from build123d import *

# Parameters (mm, degrees)
F0_W      = 80
F0_H      = 42
F1_DEPTH  = 18
F2_W      = 50
F2_H      = 42
F3_DEPTH  = 30
F4_R      = 7
F5_DEPTH  = 48
F6_R      = 15
F7_DEPTH  = 42
F9_W      = 8.9407891482
F9_H      = 20
F10_DEPTH = 29
F11_W     = 20
F11_H     = 20
F12_DEPTH = 29
F13_W     = 20
F13_H     = 20
F14_DEPTH = 29
F15_W     = 9
F15_H     = 20
F16_DEPTH = 29


with BuildPart() as f1:
    # F0 (on Front) → F1 (new body)
    with BuildSketch(Plane.XZ):
        with Locations((-5.7401350141, 5.3092095107)):
            Rectangle(F0_W, F0_H)
    extrude(amount=F1_DEPTH)

    # F2 (on face) → F3 (join)
    with BuildSketch(Plane.XZ.offset(18)):
        with Locations((-5.7401350141, 5.3092095107)):
            Rectangle(F2_W, F2_H)
    extrude(amount=F3_DEPTH)

    # F4 (on face) → F5 (cut)
    with BuildSketch(Plane.XZ.offset(48)):
        with Locations((-6.0690785758, 5.3388164379)):
            Circle(F4_R)
    extrude(amount=-F5_DEPTH, mode=Mode.SUBTRACT)

    # F6 (on face) → F7 (cut)
    with BuildSketch(Plane(origin=(0, 0, -15.6907904893), x_dir=(1, 0, 0), z_dir=(0, 0, -1))):
        with Locations((-5.7730260305, 23.694081232)):
            Circle(F6_R)
    extrude(amount=-F7_DEPTH, mode=Mode.SUBTRACT)

    # F9 (on face) → F10 (cut)
    with BuildSketch(Plane.YZ.offset(34.2598649859)):
        with Locations((-13.5296054259, 4.8190790601)):
            Rectangle(F9_W, F9_H)
    extrude(amount=-F10_DEPTH, mode=Mode.SUBTRACT)

    # F11 (on face) → F12 (cut)
    with BuildSketch(Plane.YZ.offset(19.2598649859)):
        with Locations((-28, 4.8190790601)):
            Rectangle(F11_W, F11_H)
    extrude(amount=-F12_DEPTH, mode=Mode.SUBTRACT)

    # F13 (on face) → F14 (cut)
    with BuildSketch(Plane(origin=(-30.7401350141, 0, 0), x_dir=(0, -1, 0), z_dir=(-1, 0, 0))):
        with Locations((28, 4.8190776631)):
            Rectangle(F13_W, F13_H)
    extrude(amount=-F14_DEPTH, mode=Mode.SUBTRACT)

    # F15 (on face) → F16 (cut)
    with BuildSketch(Plane(origin=(-45.7401350141, 0, 0), x_dir=(0, -1, 0), z_dir=(-1, 0, 0))):
        with Locations((13.5, 4.8190776631)):
            Rectangle(F15_W, F15_H)
    extrude(amount=-F16_DEPTH, mode=Mode.SUBTRACT)


solid = f1.part
Could you check a few things on this model? Use its own coordinates, in mm. A direction names the side the tool comes from. Round coordinates to 2 decimals unless told otherwise and drop trailing zeros. Write each loop counter-clockwise with the first axis right and the second up, starting at its lowest first coordinate (ties: lowest second). Pieces come first, ordered by that corner, then holes. Notation, with made-up numbers: (-10, -39) - (46, -39) arc R15 ccw to (46, -20) - close; hole circle Ø2 at (-26, 76.5). An arc over 180 degrees is marked (long way). Use a Markdown table: item, result.
Q1. I want a section at A-A (z = -4). List the corners of the cut face in (x, y) for me.
Output values:
| item | result |
|---|---|
| outline | (-45.74, -9) - (-16.74, -9) - (-16.74, -13.46) arc R15 cw to (5.26, -13.53) - (5.26, -9.06) - (34.26, -9.06) - (34.26, 0) - (-45.74, 0) - close; (-30.74, -48) - (19.26, -48) - (19.26, -38) - (-1.26, -38) arc R15 cw to (-10.28, -38) - (-30.74, -38) - close |
Q2. For faces 1 (the flat face through (27, -18, -10)), 2 (the flat face through (-38, -18, -10)), 3 (the flat face through (17, -21, -5.181)), 4 (the flat face through (-21, -38, 5)), 5 (the flat face through (-31, -9, 5)), which set-ups out of +Z, -Z, +X, -X, +Y, -Y let a thin tool reach every point of the face, with its end or its side?
Output values:
| item | result |
|---|---|
| face 1 | +Z, -Z, +X, -Y |
| face 2 | +Z, -Z, -X, -Y |
| face 3 | +X |
| face 4 | +X, -X |
| face 5 | -X |
Q3. I want a section at C-C (x = -14). List the corners of the cut face in (y, z) for me.
Output values:
| item | result |
|---|---|
| outline | (-48, -15.69) - (-36.24, -15.69) - (-36.24, -5.18) - (-38, -5.18) - (-38, 14.82) - (-36.24, 14.82) - (-36.24, 26.31) - (-48, 26.31) - close; (-11.15, -15.69) - (0, -15.69) - (0, 26.31) - (-11.15, 26.31) - close |
Q4. Thinking about a two-plate mould opening in X: for faces 6 (the flat face through (-16.74, -11, 5)), 7 (the flat face through (-28, -20, -5.181)), 8 (the cylindrical face through (-7.587, -43.07, -1.495)), which applies, released by +X, released by -X, zero draft, split by the parting line, or undercut?
Output values:
| item | result |
|---|---|
| face 6 | released by -X |
| face 7 | zero draft |
| face 8 | undercut |
Q5. Please list where these lines run through material, in increasing order: L1, parallel to Z at x = 11, y = -12; L2, parallel to Y at x = -26.5, z = -4; L3, parallel to X at y = -24, z = -9.
Output values:
| item | result |
|---|---|
| L1 | -15.69 to -5.18, 14.82 to 26.31 |
| L2 | -48 to -38, -9 to 0 |
| L3 | -30.74 to -20.77, 9.22 to 19.26 |
Q6. I want a section at B-B (y = -37). List the corners of the cut face in (x, z) for me, plus the area to 3 significant figures.
Output values:
| item | result |
|---|---|
| outline | (-30.74, -15.69) - (-12.7, -15.69) - (-12.7, -5.18) - (-30.74, -5.18) - close; (-30.74, 14.82) - (-12.7, 14.82) - (-12.7, 26.31) - (-30.74, 26.31) - close; (1.15, -15.69) - (19.26, -15.69) - (19.26, -5.18) - (1.15, -5.18) - close; (1.15, 14.82) - (19.26, 14.82) - (19.26, 26.31) - (1.15, 26.31) - close |
| area | 795 mm2 |
Q7. For pin 1 (3.5 mm diameter, centred on x = -38, z = 23, fed in from -Y); pin 2 (3.5 mm diameter, centred on y = -11, z = 3.5, fed in from -X); pin 3 (15 mm diameter, centred on y = -27, z = 11, fed in from +X), each with a flat end and sliding along its axis, tell me the tip position at first contact or that it passes through.
Output values:
| item | result |
|---|---|
| pin 1 | y = -18 |
| pin 2 | x = -16.74 |
| pin 3 | x = 19.26 |
Q8. I want a section at D-D (z = 9). List the corners of the cut face in (x, y) for me.
Output values:
| item | result |
|---|---|
| outline | (-45.74, -9) - (-16.74, -9) - (-16.74, -13.46) arc R15 cw to (-12.04, -10.06) - (-12.04, 0) - (-45.74, 0) - close; (-30.74, -48) - (-12.04, -48) - (-12.04, -38) - (-30.74, -38) - close; (-0.1, -48) - (19.26, -48) - (19.26, -38) - (-0.1, -38) - close; (-0.1, -9.81) arc R15 cw to (5.26, -13.53) - (5.26, -9.06) - (34.26, -9.06) - (34.26, 0) - (-0.1, 0) - close |
